```python
from build123d import *

# Parameters (mm, degrees)
SKETCH3_W           = 25.4
SKETCH3_H           = 12.7
BOSS_EXTRUDE2_DEPTH = 5.842
SKETCH4_W           = 8.466666666
SKETCH4_H           = 5.842
CUT_EXTRUDE1_DEPTH  = 16.35387456
BOSS_EXTRUDE3_DEPTH = 5.842
SKETCH10_R          = 1.27
CUT_EXTRUDE8_DEPTH  = 7.62
SKETCH12_R          = 1.27
CUT_EXTRUDE9_DEPTH  = 7.62
CUT_EXTRUDE10_DEPTH = 7.62


with BuildPart() as part:
    # Sketch3 → Boss-Extrude2 (new body)
    with BuildSketch(Plane.XY):
        Rectangle(SKETCH3_W, SKETCH3_H)
    extrude(amount=BOSS_EXTRUDE2_DEPTH)

    # Sketch4 → Cut-Extrude1 (cut, through all)
    with BuildSketch(Plane.XY.offset(5.842)):
        with Locations((0, -3.429)):
            Rectangle(SKETCH4_W, SKETCH4_H)
    extrude(amount=-CUT_EXTRUDE1_DEPTH, mode=Mode.SUBTRACT)

    # Sketch5 → Boss-Extrude3 (add)
    with BuildSketch(Plane.XY.offset(5.842)):
        with BuildLine():
            Line((0, 44.45), (27.164431218, 44.45))
            add(Edge.make_bspline(
                [(12.7, 6.35), (11.748773867, 28.101932144), (27.164431218, 44.45)],
                knots=[0, 0, 0, 1, 1, 1], degree=2))
            Line((12.7, 6.35), (-12.7, 6.35))
            add(Edge.make_bspline(
                [(-12.7, 6.35), (-10.61981434, 26.757908534), (0, 44.45)],
                knots=[0, 0, 0, 1, 1, 1], degree=2))
        make_face()
    extrude(amount=-BOSS_EXTRUDE3_DEPTH)

    # Sketch10 → Cut-Extrude8 (cut)
    with BuildSketch(Plane.XY.offset(5.842)):
        with Locations((7.264189007, 6.800526763)):
            Circle(SKETCH10_R)
    extrude(amount=-CUT_EXTRUDE8_DEPTH, mode=Mode.SUBTRACT)

    # Sketch12 → Cut-Extrude9 (cut)
    with BuildSketch(Plane.XY.offset(5.842)):
        with Locations((5.572598549, 28.091285842)):
            Circle(SKETCH12_R)
        with Locations((6.546271927, 21.532393633)):
            Circle(SKETCH12_R)
        with Locations((7.173302087, 13.821975993)):
            Circle(SKETCH12_R)
        with Locations((2.529205303, 40.659348041)):
            Circle(SKETCH12_R)
        with Locations((4.243902878, 34.397725849)):
            Circle(SKETCH12_R)
    extrude(amount=-CUT_EXTRUDE9_DEPTH, mode=Mode.SUBTRACT)

    # Sketch13 → Cut-Extrude10 (cut)
    with BuildSketch(Plane.XY.offset(5.842)):
        Polygon((-2.774085904, 26.946129085), (-7.675131543, 7.341946529), (1.582399109, 7.341946529), align=None)
        Polygon((10.172842992, 40.693017541), (12.474681541, 30.334744073), (19.066310112, 40.693017541), align=None)
    extrude(amount=-CUT_EXTRUDE10_DEPTH, mode=Mode.SUBTRACT)


solid = part.part
```
Source: CAD feature listing. Evaluate the final solid. Frame: model axes, mm. A direction names the side the tool comes from. Round coordinates to 2 decimals unless told otherwise and drop trailing zeros. Use CSV: the item, a comma, the result in double quotes.
Q1. Ray query, line 1 along Y through (x, z) = (6.5, 3.05); line 2 along X through (y, z) = (2.5, 3.2); line 3 along X through (y, z) = (22, 1). Return the intervals inside material, ascending.
Reported:
line 1,"-6.35 to 5.79, 7.81 to 12.75, 14.9 to 20.26, 22.8 to 27.22, 28.96 to 44.45"
line 2,"-12.7 to 12.7"
line 3,"-9.74 to -4.01, -1.67 to 5.37, 7.73 to 14.31"
Q2. Reachability of faces 1 (the flat face through (-4.233, -3, 3)), 2 (the flat face through (13, 44.45, 3)), 3 (the flat face through (-5.19, 17.28, 2.96)) from +Z, -Z, +X, -X, +Y, -Y: full face, straight path, thin tool, end or side. Return the list, or none.
Reported:
face 1,"+Z, -Z, -Y"
face 2,"+Z, -Z, +X, -X, +Y"
face 3,"+Z, -Z"
Q3. Pin query (flat end, axial travel): pin 1 Ø3 at (x, z) = (-2.5, 3.5) entering from +Y (3 decimals); pin 2 Ø3 at (y, z) = (-1.5, 2) entering from +X; pin 3 Ø1.8 at (x, z) = (2, 1.5) entering from -Y. Return the tip coordinate at first contact, or that it passes through.
Reported:
pin 1,"y = 42.745"
pin 2,"x = 12.7"
pin 3,"y = -0.51"
Q4. Mould query, pull axis X, two halves, no side actions, for faces 4 (the flat face through (12.7, 0, 3)), 5 (the flat face through (15, 40.693, 3)), 6 (the flat face through (8, -6.35, 3)). Classes: pulls with the +X half, pulls with the -X half, needs draft (parallel to the pull), parting line crosses it, or undercut.
Reported:
face 4,"pulls with the +X half"
face 5,"undercut"
face 6,"needs draft"
Q5. Section query A-A, the plane z = 3.3. Give the number of separate pieces and of enclosed holes in the cut face, then the cut area to 3 significant figures.
Reported:
separate pieces,"1"
enclosed holes,"8"
area,"1,050 mm^2"
